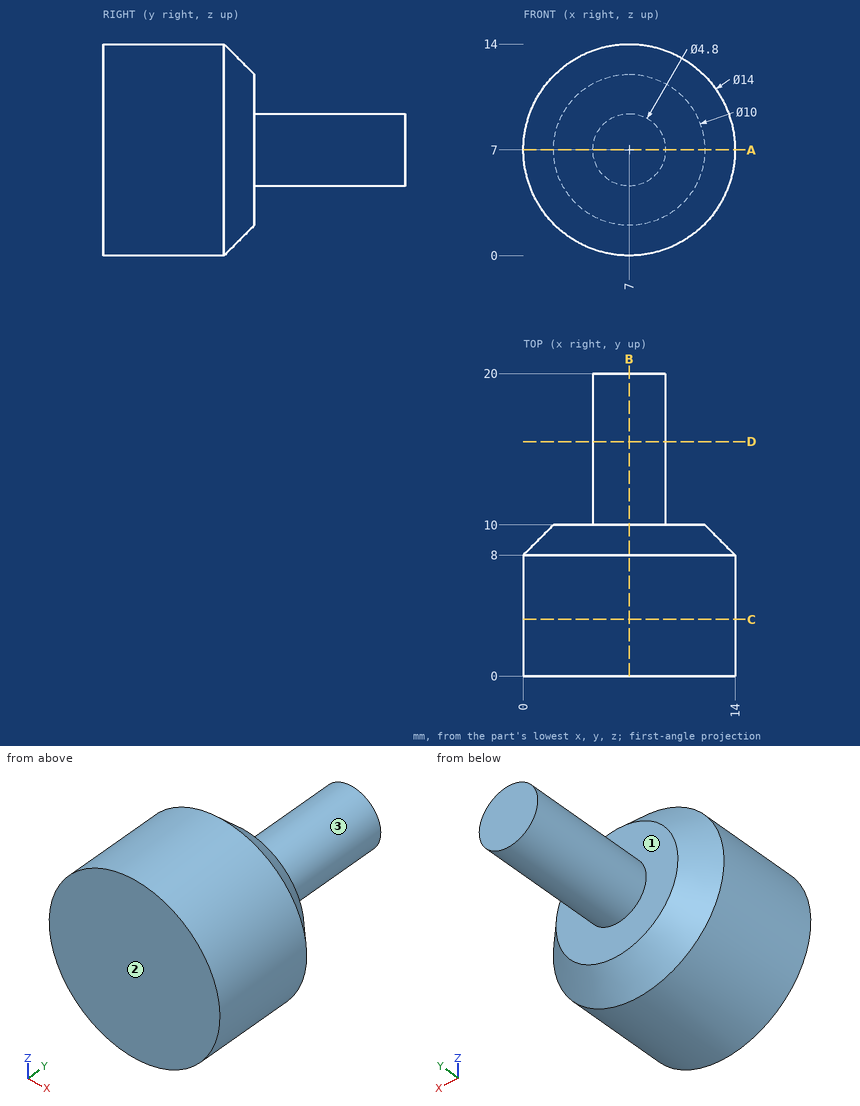
Input: dimensioned drawing with shaded views. Units: mm. Origin: part minimum x, y, z. Round coordinates to 2 decimals unless told otherwise and drop trailing zeros. Order: outer loops, then holes, each group sorted by start corner. A loop starts at its lowest first (then second) coordinate and runs counter-clockwise, first axis right, second up. Notation, with made-up numbers: (65, -13) -> (85, -13) arc R21 cw to (85, 18) -> close; hole circle Ø4 at (-26, 22.25). An arc over 180 degrees is marked (long way). Put each result on its own line as item: value. Start each with the question number.
Q1. First-contact query: pin 1 (5 mm diameter, centred on y = 6, z = 4, fed in from +X); pin 2 (2 mm diameter, centred on y = 13, z = 7.5, fed in from +X); pin 3 (1.5 mm diameter, centred on y = 9.5, z = 12, fed in from -X); pin 4 (6 mm diameter, centred on y = 7, z = 9.5, fed in from -X). Flat tips, straight axial feed; report the tip coordinate or a pass-through.
Q2. Section D-D on y = 15.5. Return the cut outline in (x, z).
Q3. Line query: probe 1 along Y at (x, z) = (11, 9.5); probe 2 along Z at (x, y) = (7.5, 2.5); probe 3 along X at (y, z) = (6.75, 4.75). Output: solid intervals per line, ascending.
Q4. Section A-A on z = 7. Return the cut outline in (x, y).
Q5. Section C-C on y = 3.75. Return the cut outline in (x, z).
Q6. Section B-B on x = 7. Return the cut outline in (y, z), and give its area (3 significant figures).
Q7. Pull-direction query (Y, two-part tool) for the marked faces 1, 2 and 3; classes: +Y half, -Y half, draft (parallel to the pull), parting line (faces both ways), or undercut.
Ans:
1. pin 1: stops at x = 13.98
1. pin 2: stops at x = 9.4
1. pin 3: stops at x = 2.94
1. pin 4: stops at x = 0
2. outline: circle Ø4.8 at (7, 7)
3. probe 1: y = 0 to 10
3. probe 2: z = 0.02 to 13.98
3. probe 3: x = 0.37 to 13.63
4. outline: (0, 0) -> (14, 0) -> (14, 8) -> (12, 10) -> (9.4, 10) -> (9.4, 20) -> (4.6, 20) -> (4.6, 10) -> (2, 10) -> (0, 8) -> close
5. outline: circle Ø14 at (7, 7)
6. outline: (0, 0) -> (8, 0) -> (10, 2) -> (10, 4.6) -> (20, 4.6) -> (20, 9.4) -> (10, 9.4) -> (10, 12) -> (8, 14) -> (0, 14) -> close
6. area: 184 mm2
7. face 1: +Y half
7. face 2: -Y half
7. face 3: draft
